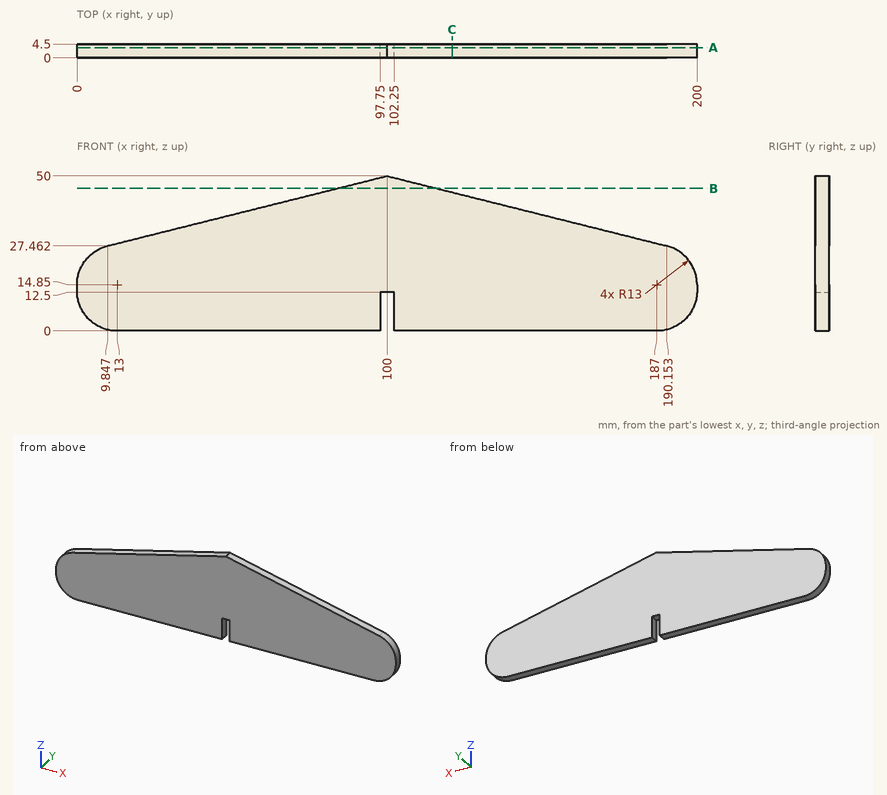
Verification items for this drawing (mm, ordinates from the low corner). Give positions to 0.01 mm unless a question says otherwise; leave off trailing zeros. Loops run counter-clockwise (first coordinate to the right, second up) from the corner with the lowest first, then second, coordinate; pieces in that order, holes last. Notation, with made-up numbers: M 15.25,4.5 L 60.25,4.5 A14 ccw 60.25,12.5 Z; hole C 34,67 d2. An arc over 180 degrees is marked long. Answer in a Markdown table with one row per item.
1) Cross-section at A-A (y = 3.35). Enter the section's corners in (x, z), plus the area to 3 significant figures.
Solutions:
| item | result |
|---|---|
| outline | M 0,13 A13 ccw 13,0 L 97.75,0 L 97.75,12.5 L 102.25,12.5 L 102.25,0 L 187,0 A13 ccw 200,13 L 200,14.85 A13 ccw 190.15,27.46 L 100,50 L 9.85,27.46 A13 ccw 0,14.85 Z |
| area | 7,330 mm^2 |
2) Thickness scan on line 1 (X direction, y = 4.25, z = 5.5); line 2 (X direction, y = 3.75, z = 8); line 3 (Z direction, x = 99, y = 0.75). Record the ranges inside material, lowest first.
Solutions:
| item | result |
|---|---|
| line 1 | x = 2.38 to 97.75, 102.25 to 197.62 |
| line 2 | x = 1 to 97.75, 102.25 to 199 |
| line 3 | z = 12.5 to 49.75 |
3) Cross-section at B-B (z = 46). Enter the section's corners in (x, y), plus the area to 3 significant figures.
Solutions:
| item | result |
|---|---|
| outline | M 84,0 L 116,0 L 116,4.5 L 84,4.5 Z |
| area | 144 mm^2 |
4) Depth check by flat-ended pin: pin 1 (2 mm diameter, centred on x = 101, y = 3, fed in from -Z). Enter the tip coordinate at first touch or a pass-through.
Solutions:
| item | result |
|---|---|
| pin 1 | stops at z = 12.5 |
5) Cross-section at C-C (x = 121). Enter the section's corners in (y, z), plus the area to 3 significant figures.
Solutions:
| item | result |
|---|---|
| outline | M 0,0 L 4.5,0 L 4.5,44.75 L 0,44.75 Z |
| area | 201 mm^2 |
